```python
from build123d import *

# Parameters (mm, degrees)
F0_W     = 205.74
F0_H     = 205.74
F0_R     = 46.101
F1_DEPTH = 64.516
F2_W     = 161.544
F2_H     = 161.544
F2_R     = 46.101
F3_DEPTH = 58.42


with BuildPart() as f1:
    # F0 (on Front) → F1 (new body)
    with BuildSketch(Plane.XZ):
        with Locations((-59.400756, -2.085568)):
            Rectangle(F0_W, F0_H)
        with Locations((-59.400756, -2.085568)):
            Circle(F0_R, mode=Mode.SUBTRACT)
    extrude(amount=F1_DEPTH)

    # F2 (on face) → F3 (cut)
    with BuildSketch(Plane.XZ.offset(64.516)):
        with Locations((-59.400756, -2.085568)):
            Rectangle(F2_W, F2_H)
        with Locations((-59.400756, -2.085568)):
            Circle(F2_R, mode=Mode.SUBTRACT)
    extrude(amount=-F3_DEPTH, mode=Mode.SUBTRACT)


solid = f1.part
```
Check sheet for the modelled part. Datum: model origin and axes. Units: mm. A direction names the side the tool comes from. Coordinates: 2 decimals unless noted, no trailing zeros. Order: outer loops, then holes, each group sorted by start corner. A loop starts at its lowest first (then second) coordinate and runs counter-clockwise, first axis right, second up. Notation, with made-up numbers: M 76,72.25 L 107,72.25 A9 ccw 107,81.25 Z; hole C 68,-14.5 d4. An arc over 180 degrees is marked long. Write each question's results on one line, items separated by ' | '. Start each with the question number.
1. Access from +Z, -Z, +X, -X, +Y, -Y to the whole of each face (thin tool, end or side, straight path). Record for faces 4 (the face through (-61, -36, 78.686)), 5 (the face through (-61, 0, 45)).
2. Mould release check, pull along X, two halves, no side actions. Record for faces 1 (the face through (-162.271, -32, -4)), 2 (the face through (-61, -32, 100.784)), 3 (the face through (-96, -6.096, 35)): +X half, -X half, draft (parallel to the pull), parting line (faces both ways), or undercut.
3. Material ranges on probe 1 along Z at (x, y) = (-68, -39.5); probe 2 along X at (y, z) = (-47, -75); probe 3 along Y at (x, z) = (-134.5, -13), recorded low to high.
4. Cross-section at B-B on x = -23. Record the cut outline in (y, z), and give its area (3 significant figures).
5. Go/stop test with a flat-tipped pin: P1, Ø12, axis at x = -6, z = -15.5, coming from the -Y side. Record where the tip stops, or that it passes through.
6. Cross-section at D-D on x = -125. Record the cut outline in (y, z), and give its area (3 significant figures).
7. Cross-section at C-C on z = 30.5. Record the cut outline in (x, y), and give its area (3 significant figures).
8. Cross-section at A-A on y = -23. Record the cut outline in (x, z), and give its area (3 significant figures).
Checks:
1) face 4: -Y | face 5: +Z, -Z, +X, -X, +Y
2) face 1: -X half | face 2: draft | face 3: undercut
3) probe 1: z = -104.96 to -82.86, 78.69 to 100.78 | probe 2: x = -162.27 to -140.17, 21.37 to 43.47 | probe 3: y = -6.1 to 0
4) outline: M -64.52,-104.96 L 0,-104.96 L 0,-30.37 L -6.1,-30.37 L -6.1,-82.86 L -64.52,-82.86 Z; M -64.52,78.69 L -6.1,78.69 L -6.1,26.2 L 0,26.2 L 0,100.78 L -64.52,100.78 Z | area: 3,490 mm²
5) P1: stops at y = -6.1
6) outline: M -64.52,-104.96 L 0,-104.96 L 0,100.78 L -64.52,100.78 L -64.52,78.69 L -6.1,78.69 L -6.1,-82.86 L -64.52,-82.86 Z | area: 3,840 mm²
7) outline: M -162.27,-64.52 L -140.17,-64.52 L -140.17,-6.1 L -92.01,-6.1 L -92.01,0 L -162.27,0 Z; M -26.79,-6.1 L 21.37,-6.1 L 21.37,-64.52 L 43.47,-64.52 L 43.47,0 L -26.79,0 Z | area: 3,440 mm²
8) outline: M -162.27,-104.96 L 43.47,-104.96 L 43.47,100.78 L -162.27,100.78 Z; hole M -140.17,-82.86 L 21.37,-82.86 L 21.37,78.69 L -140.17,78.69 Z | area: 16,200 mm²
